CAD build for the part. Positions are in the model's coordinates, mm. A direction names the side the tool comes from. Give positions to 0.01 mm unless a question says otherwise; leave off trailing zeros. Write each loop counter-clockwise with the first axis right and the second up, starting at its lowest first coordinate (ties: lowest second). Pieces come first, ordered by that corner, then holes. Notation, with made-up numbers: (28, 26.25) -> (54, 26.25) arc R16 ccw to (54, 53.25) -> close; hole circle Ø3 at (70, 7). An arc over 180 degrees is marked (long way). Answer as a JSON object with one key per item and string values.
```python
from build123d import *

# Parameters (mm, degrees)
F1_DEPTH = 20
F2_R     = 4
F2_R_2   = 1.5
F3_DEPTH = 4
F4_DEPTH = 25


with BuildPart() as f1:
    # F0 (on Top) → F1 (new body)
    with BuildSketch(Plane.XY):
        with BuildLine():
            Line((-20, 0), (0, 0))
            Line((0, 0), (0, 3))
            Line((0, 3), (-23, 3))
            Line((-23, 3), (-23, -21.2))
            Line((-23, -21.2), (-12.4687010187, -21.2))
            ThreePointArc((-12.4687010187, -21.2), (-7.7051657034, -18.9662531166), (-2.5, -18.2))
            Line((-2.5, -18.2), (-20, -18.2))
            Line((-20, -18.2), (-20, 0))
        make_face()
        with BuildLine():
            ThreePointArc((7.4687010187, -21.2), (2.7051657034, -18.9662531166), (-2.5, -18.2))
            ThreePointArc((-2.5, -18.2), (-7.7051657034, -18.9662531166), (-12.4687010187, -21.2))
            Line((-12.4687010187, -21.2), (-2.5000000655, -21.2))
            Line((-2.5000000655, -21.2), (7.4687010187, -21.2))
        make_face()
        with BuildLine():
            Line((15, -18.2), (-2.5, -18.2))
            ThreePointArc((-2.5, -18.2), (2.7051657034, -18.9662531166), (7.4687010187, -21.2))
            Line((7.4687010187, -21.2), (15, -21.2))
            Line((15, -21.2), (15, -18.2))
        make_face()
        with BuildLine():
            ThreePointArc((12.5, -26.2), (10.2322035658, -23.4505954339), (7.4687010187, -21.2))
            Line((7.4687010187, -21.2), (-2.5000000655, -21.2))
            ThreePointArc((-2.5000000655, -21.2), (3.6364688244, -22.5066773559), (8.7082558857, -26.2))
            ThreePointArc((8.7082558857, -26.2), (3.6364688543, -29.8933226308), (-2.5, -31.2))
            Line((-2.5, -31.2), (3.1142186431, -33.3053319912))
            ThreePointArc((3.1142186431, -33.3053319912), (8.4021987802, -30.538748835), (12.5, -26.2))
        make_face()
        with BuildLine():
            ThreePointArc((-2.5, -34.2), (0.3425288837, -33.974930751), (3.1142186431, -33.3053319912))
            Line((3.1142186431, -33.3053319912), (-2.5, -31.2))
            Line((-2.5, -31.2), (-8.1142186431, -33.3053319912))
            ThreePointArc((-8.1142186431, -33.3053319912), (-5.3425288837, -33.974930751), (-2.5, -34.2))
        make_face()
        with BuildLine():
            Line((-2.5000000655, -21.2), (-12.4687010187, -21.2))
            ThreePointArc((-12.4687010187, -21.2), (-15.2322035658, -23.4505954339), (-17.5, -26.2))
            ThreePointArc((-17.5, -26.2), (-13.4021987802, -30.538748835), (-8.1142186431, -33.3053319912))
            Line((-8.1142186431, -33.3053319912), (-2.5, -31.2))
            ThreePointArc((-2.5, -31.2), (-8.6364688543, -29.8933226308), (-13.7082558857, -26.2))
            ThreePointArc((-13.7082558857, -26.2), (-8.6364688842, -22.5066773825), (-2.5000000655, -21.2))
        make_face()
        with BuildLine():
            ThreePointArc((-2.5, -34.2), (-5.3425288837, -33.974930751), (-8.1142186431, -33.3053319912))
            Line((-8.1142186431, -33.3053319912), (-10.5, -34.2))
            Line((-10.5, -34.2), (-2.5, -34.2))
        make_face()
        with BuildLine():
            Line((5.5, -34.2), (3.1142186431, -33.3053319912))
            ThreePointArc((3.1142186431, -33.3053319912), (0.3425288837, -33.974930751), (-2.5, -34.2))
            Line((-2.5, -34.2), (5.5, -34.2))
        make_face()
    extrude(amount=F1_DEPTH)

    # F2 (on face) → F3 (cut)
    with BuildSketch(Plane.XZ.offset(34.2)):
        with Locations((-2.5, 10)):
            Circle(F2_R)
        with Locations((-2.5, 10)):
            Circle(F2_R_2, mode=Mode.SUBTRACT)
    extrude(amount=-F3_DEPTH, mode=Mode.SUBTRACT)

    # F4 (cut): a face of the model
    f4_faces = [f1.faces().sort_by_distance(p)[0] for p in [
        (-2.5, -34.2, 10),
    ]]
    extrude(f4_faces, amount=-F4_DEPTH, mode=Mode.SUBTRACT)


solid = f1.part
```
1) Slice it at D-D (z = 14.75). List the corners of the cut face in (x, y) (1 decimal).
Model answer:
{"outline": "(-23, -21.2) -> (-12.5, -21.2) arc R18.1 ccw to (-17.5, -26.2) arc R18.1 ccw to (-8.1, -33.3) -> (-10.5, -34.2) -> (5.5, -34.2) -> (3.1, -33.3) arc R18.1 ccw to (12.5, -26.2) arc R18.1 ccw to (7.5, -21.2) -> (15, -21.2) -> (15, -18.2) -> (-20, -18.2) -> (-20, 0) -> (0, 0) -> (0, 3) -> (-23, 3) -> close; hole (-13.7, -26.2) arc R15.1 ccw to (8.7, -26.2) arc R15.1 ccw to start"}
2) 3-axis set-ups, long thin cutter, end or side, ignore diameter. For faces 1 (the cylindrical face through (-2.7, -21.2, 12.1)), 2 (the flat face through (-10, 0, 10)), 3 (the cylindrical face through (-2.825, -19.76, 8.536)), 4 (the flat face through (-18, -21.2, 10)): which of +Z, -Z, +X, -X, +Y, -Y reach the whole face in a straight line?
Model answer:
{"face 1": "+Z, -Z", "face 2": "+Z, -Z, +X", "face 3": "-Y", "face 4": "+Z, -Z, -X"}
3) Wall check: probe 1 along X at (y, z) = (-20.35, 10); probe 2 along Z at (x, y) = (-2.5, -18.8); probe 3 along Y at (x, z) = (-14.5, 4.75). Give the ranges that are in metal, low to high.
Model answer:
{"probe 1": "x = -23 to -4, -1 to 15", "probe 2": "z = 0 to 8.5, 11.5 to 20", "probe 3": "y = -29.64 to -22.76, -21.2 to -18.2, 0 to 3"}
4) Slice it at B-B (z = 10). List the corners of the cut face in (x, y) (1 decimal).
Model answer:
{"outline": "(-23, -21.2) -> (-12.5, -21.2) arc R18.1 ccw to (-17.5, -26.2) arc R18.1 ccw to (-8.1, -33.3) -> (-10.5, -34.2) -> (-6.5, -34.2) -> (-6.5, -30.7) arc R15.1 cw to (-13.7, -26.2) arc R15.1 cw to (-4, -21.3) -> (-4, -18.2) -> (-20, -18.2) -> (-20, 0) -> (0, 0) -> (0, 3) -> (-23, 3) -> close; (-1, -21.3) arc R15.1 cw to (8.7, -26.2) arc R15.1 cw to (1.5, -30.7) -> (1.5, -34.2) -> (5.5, -34.2) -> (3.1, -33.3) arc R18.1 ccw to (12.5, -26.2) arc R18.1 ccw to (7.5, -21.2) -> (15, -21.2) -> (15, -18.2) -> (-1, -18.2) -> close"}
5) Mould opens along Y. For faces 5 (the flat face through (-20, -9, 10)), 6 (the flat face through (-11, 3, 10)), 7 (the flat face through (0, 1, 10)) say: released by +Y, released by -Y, zero draft, split by the parting line, or undercut.
Model answer:
{"face 5": "undercut", "face 6": "released by +Y", "face 7": "zero draft"}
6) Slice it at C-C (x = 10.5). List the corners of the cut face in (y, z), then the cut area to 3 significant figures.
Model answer:
{"outline": "(-28.68, 0) -> (-23.72, 0) -> (-23.72, 20) -> (-28.68, 20) -> close; (-21.2, 0) -> (-18.2, 0) -> (-18.2, 20) -> (-21.2, 20) -> close", "area": "159 mm2"}
7) Slice it at A-A (x = -2.5). List the corners of the cut face in (y, z).
Model answer:
{"outline": "(-34.2, 0) -> (-31.2, 0) -> (-31.2, 6) -> (-34.2, 6) -> close; (-34.2, 14) -> (-31.2, 14) -> (-31.2, 20) -> (-34.2, 20) -> close; (-21.2, 0) -> (-18.2, 0) -> (-18.2, 8.5) -> (-21.2, 8.5) -> close; (-21.2, 11.5) -> (-18.2, 11.5) -> (-18.2, 20) -> (-21.2, 20) -> close; (0, 0) -> (3, 0) -> (3, 20) -> (0, 20) -> close"}
8) Pin check, flat tips, straight feed: pin 1 (8.5 mm diameter, centred on x = 12.5, z = 8.5, fed in from -Y); pin 2 (6 mm diameter, centred on x = -15, z = 8, fed in from -Y); pin 3 (1.5 mm diameter, centred on y = -26, z = 7, fed in from +X). Stop position of each tip, or through.
Model answer:
{"pin 1": "stops at y = -30.65", "pin 2": "stops at y = -31.5", "pin 3": "stops at x = 12.5"}
